```python
from build123d import *

# Parameters (mm, degrees)
F1_DEPTH = 8
F2_W     = 5.8
F2_H     = 8
F3_DEPTH = 8
F4_R     = 0.1


# Not quite as in the source:
# - a feature names something its author has since deleted; it is built from what else it names


with BuildPart() as f1:
    # F0 (on Top) → F1 (new body)
    with BuildSketch(Plane.XY):
        Polygon((-16.1652290315, 5.6598789893), (-45.1652290315, 5.6598789893), (-45.1652290315, 4.1598789893), (-46.7652290315, 4.1598789893), (-46.7652290315, 5.6598789893), (-48.1652290315, 5.6598789893), (-48.1652290315, -0.1401210107), (-46.7652290315, -0.1401210107), (-46.7652290315, 1.3598789893), (-45.1652290315, 1.3598789893), (-45.1652290315, -0.1401210107), (-16.1652290315, -0.1401210107), align=None)
    extrude(amount=F1_DEPTH)

    # F2 (on face) → F3 (cut)
    with BuildSketch(Plane.YZ.offset(-16.1652290315)):
        with Locations((2.7598789893, 4)):
            Rectangle(F2_W, F2_H)
        Polygon((4.7098789893, 0.05), (2.7598789893, 0.05), (0.8098789893, 0.05), (0.8098789893, 4), (0.8098789893, 7.95), (2.7598789893, 7.95), (4.7098789893, 7.95), (4.7098789893, 4), align=None, mode=Mode.SUBTRACT)
    extrude(amount=-F3_DEPTH, mode=Mode.SUBTRACT)

    # F4
    f4_edges = [f1.edges().sort_by_distance(p)[0] for p in [
        (-46.765229, -0.140121, 4),
        (-46.765229, 1.359879, 4),
        (-46.765229, 4.159879, 4),
        (-46.765229, 5.659879, 4),
        (-48.165229, 5.659879, 4),
        (-48.165229, -0.140121, 4),
        (-45.165229, -0.140121, 4),
        (-45.165229, 5.659879, 4),
        (-45.165229, 4.159879, 4),
        (-45.165229, 1.359879, 4),
    ]]
    fillet(f4_edges, radius=F4_R)


solid = f1.part
```
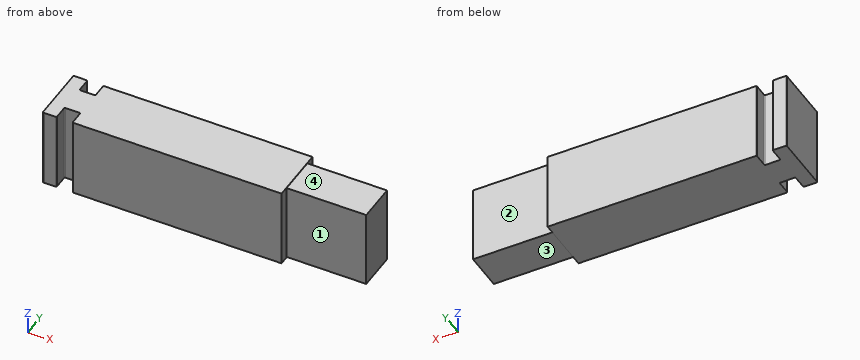
Could you check a few things on this model? Use its own coordinates, in mm. Face numbers are marked on the shaded views. A direction names the side the tool comes from. Round coordinates to 2 decimals unless told otherwise and drop trailing zeros. Loops run counter-clockwise (first coordinate to the right, second up) from the corner with the lowest first, then second, coordinate; pieces in that order, holes last.
Q1. I want a section at B-B (z = 0.75). Write out the boundary of the cut face in (x, y).
Q2. On a 3-axis mill with a long thin cutter (end or side, diameter ignored), from which of +Z, -Z, +X, -X, +Y, -Y can I reach the whole of each face in a straight line? I mean the marked faces 1, 2, 3 and 4. Say none if no direction works.
Q3. I want a section at C-C (x = -19). Write out the boundary of the cut face in (y, z).
Q4. For P1, Ø1.2, axis at x = -20.5, y = 3.5, coming from the -Z side; P2, Ø2, axis at x = -19, y = 2, coming from the +Z side; P3, Ø2.5, axis at x = -19, z = 3.5, coming from the +Y side, each with a flat end and sliding along its axis, tell me the tip position at first contact or that it passes through.
Q5. Please list where these lines run through material, in increasing order: L1, parallel to X at y = 0.4, z = 1; L2, parallel to Z at x = -21, y = 2.1; L3, parallel to Y at x = -24, z = 2.
Q6. I want a section at A-A (y = 0.5). Write out the boundary of the cut face in (x, z).
Answer below:
1. outline: (-48.17, -0.04) arc R0.1 ccw to (-48.07, -0.14) - (-46.87, -0.14) arc R0.1 ccw to (-46.77, -0.04) - (-46.77, 1.26) arc R0.1 cw to (-46.67, 1.36) - (-45.27, 1.36) arc R0.1 cw to (-45.17, 1.26) - (-45.17, -0.04) arc R0.1 ccw to (-45.07, -0.14) - (-24.17, -0.14) - (-24.17, 0.81) - (-16.17, 0.81) - (-16.17, 4.71) - (-24.17, 4.71) - (-24.17, 5.66) - (-45.07, 5.66) arc R0.1 ccw to (-45.17, 5.56) - (-45.17, 4.26) arc R0.1 cw to (-45.27, 4.16) - (-46.67, 4.16) arc R0.1 cw to (-46.77, 4.26) - (-46.77, 5.56) arc R0.1 ccw to (-46.87, 5.66) - (-48.07, 5.66) arc R0.1 ccw to (-48.17, 5.56) - close
2. face 1: +Z, -Z, +X, -Y
2. face 2: +Z, -Z, +X, +Y
2. face 3: -Z, +X, +Y, -Y
2. face 4: +Z, +X, +Y, -Y
3. outline: (0.81, 0.05) - (4.71, 0.05) - (4.71, 7.95) - (0.81, 7.95) - close
4. P1: stops at z = 0.05
4. P2: stops at z = 7.95
4. P3: stops at y = 4.71
5. L1: x = -48.17 to -46.77, -45.17 to -24.17
5. L2: z = 0.05 to 7.95
5. L3: y = 0.81 to 4.71
6. outline: (-48.17, 0) - (-46.77, 0) - (-46.77, 8) - (-48.17, 8) - close; (-45.17, 0) - (-24.17, 0) - (-24.17, 8) - (-45.17, 8) - close
